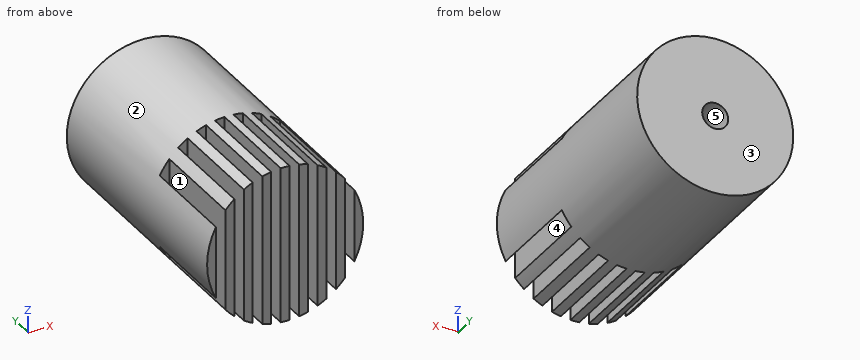
```python
from build123d import *

# Parameters (mm, degrees)
ESQUISSE1_R             = 38.1
BOSS_EXTRU_1_DEPTH      = 63.5
ESQUISSE2_R             = 6.35
ENL_V_MAT_EXTRU_1_DEPTH = 17.78
ESQUISSE3_R             = 25.4
ENL_V_MAT_EXTRU_2_DEPTH = 50.8
ESQUISSE4_W             = 4.66725
ESQUISSE4_H             = 76.2
ENL_V_MAT_EXTRU_3_DEPTH = 50.8


with BuildPart() as part:
    # Esquisse1 → Boss.-Extru.1 (new, symmetric)
    with BuildSketch(Plane(origin=(0, 0, 0), x_dir=(1, 0, 0), z_dir=(0, 1, 0))):
        with Locations(Location((0, 0, 0), (0, 0, 270))):
            Circle(ESQUISSE1_R)
    extrude(amount=BOSS_EXTRU_1_DEPTH, both=True)

    # Esquisse2 → Enlèv. mat.-Extru.1 (cut)
    with BuildSketch(Plane(origin=(0, 63.5, 0), x_dir=(1, 0, 0), z_dir=(0, 1, 0))):
        with Locations(Location((0, 0, 0), (0, 0, 270))):
            Circle(ESQUISSE2_R)
    extrude(amount=-ENL_V_MAT_EXTRU_1_DEPTH, mode=Mode.SUBTRACT)

    # Esquisse3 → Enlèv. mat.-Extru.2 (cut)
    with BuildSketch(Plane(origin=(0, 45.72, 0), x_dir=(1, 0, 0), z_dir=(0, 1, 0))):
        with Locations(Location((0, 0, 0), (0, 0, 270))):
            Circle(ESQUISSE3_R)
    extrude(amount=-ENL_V_MAT_EXTRU_2_DEPTH, mode=Mode.SUBTRACT)

    # Esquisse4 → Enlèv. mat.-Extru.3 (cut)
    with BuildSketch(Plane.XZ.offset(63.5)):
        with Locations((22.458375, 0)):
            Rectangle(ESQUISSE4_W, ESQUISSE4_H)
        with Locations((31.448375, 0)):
            Rectangle(ESQUISSE4_W, ESQUISSE4_H)
        with Locations((13.468375, 0)):
            Rectangle(ESQUISSE4_W, ESQUISSE4_H)
        with Locations((4.478375, 0)):
            Rectangle(ESQUISSE4_W, ESQUISSE4_H)
        with Locations((-4.511625, 0)):
            Rectangle(ESQUISSE4_W, ESQUISSE4_H)
        with Locations((-13.501625, 0)):
            Rectangle(ESQUISSE4_W, ESQUISSE4_H)
        with Locations((-22.491625, 0)):
            Rectangle(ESQUISSE4_W, ESQUISSE4_H)
        with Locations((-31.481625, 0)):
            Rectangle(ESQUISSE4_W, ESQUISSE4_H)
    extrude(amount=-ENL_V_MAT_EXTRU_3_DEPTH, mode=Mode.SUBTRACT)


solid = part.part
```
Design review of the part built by this model. Coordinates are the model's own, in mm. Face numbers are marked on the shaded views. A direction names the side the tool comes from. Coordinates: 2 decimals unless noted, no trailing zeros. Order: outer loops, then holes, each group sorted by start corner. A loop starts at its lowest first (then second) coordinate and runs counter-clockwise, first axis right, second up. Notation, with made-up numbers: M 85,-31 L 115,-31 A22 cw 115,-1 Z; hole C -34.5,29.25 d5. An arc over 180 degrees is marked long. Answer as a JSON object with one key per item and string values. Group by question number.
1) For pin 1 (3 mm diameter, centred on y = 36.5, z = 29.5, fed in from -X); pin 2 (2.5 mm diameter, centred on x = 23.5, z = -4, fed in from -Y); pin 3 (12 mm diameter, centred on y = 28, z = 4.5, fed in from -X), all flat-tipped, find the tip position at first contact; note any pin that passes through.
2) Tool access review of the marked faces 4 and 5: name each direction out of +Z, -Z, +X, -X, +Y, -Y from which nothing blocks a thin tool from reaching the whole face with its end or side.
3) Wall thickness on L1, parallel to X at y = 16.5, z = 0; L2, parallel to X at y = 59.75, z = 0; L3, parallel to Y at x = -2, z = 17.5: over which ranges is each line inside the solid? List them lowest first.
4) Add section D-D, the plane y = 35. Write out the cut boundary in (x, z), then the cut area to 3 significant figures.
5) Add section A-A, the plane y = -27. Count the separate pieces of the cut face and the enclosed holes in it, then the cut area to 3 significant figures.
6) Add section B-B, the plane x = 0. Write out the cut boundary in (y, z).
7) Add section C-C, the plane x = 14. Write out the cut boundary in (y, z).
8) Mouldability with a two-part tool opening along X and no side actions: class the marked faces 1, 2 and 3 as pulls with the +X half, pulls with the -X half, needs draft (parallel to the pull), parting line crosses it, or undercut.
Computed values:
{
 "1": {"pin 1": "stops at x = -25.84", "pin 2": "stops at y = -12.7", "pin 3": "stops at x = -38.1"},
 "2": {"face 4": "+Z, -Z, -Y", "face 5": "+Y"},
 "3": {"L1": "x = -38.1 to -25.4, 25.4 to 38.1", "L2": "x = -38.1 to -6.35, 6.35 to 38.1", "L3": "y = -63.5 to -5.08, 45.72 to 63.5"},
 "4": {"outline": "C 0,0 d76.2; hole C 0,0 d50.8", "area": "2,530 mm^2"},
 "5": {"separate pieces": "9", "enclosed holes": "0", "area": "2,220 mm^2"},
 "6": {"outline": "M -63.5,-38.1 L 63.5,-38.1 L 63.5,-6.35 L 45.72,-6.35 L 45.72,-25.4 L -5.08,-25.4 L -5.08,25.4 L 45.72,25.4 L 45.72,6.35 L 63.5,6.35 L 63.5,38.1 L -63.5,38.1 Z"},
 "7": {"outline": "M -12.7,-35.43 L 63.5,-35.43 L 63.5,35.43 L -12.7,35.43 Z; hole M -5.08,-21.19 L 45.72,-21.19 L 45.72,21.19 L -5.08,21.19 Z"},
 "8": {"face 1": "undercut", "face 2": "parting line crosses it", "face 3": "needs draft"}
}
